Can you work these out from the drawing? Everything is in mm from the part's minimum corner. Coordinates: 2 decimals unless noted, no trailing zeros. Write each loop counter-clockwise with the first axis right and the second up, starting at its lowest first coordinate (ties: lowest second). Pieces come first, ordered by that corner, then holes. Notation, with made-up numbers: M -3,64 L 11,64 A22 ccw 11,81 Z; hole C 21.25,62.25 d11. An arc over 180 degrees is marked long. Write each question's results on one line, items separated by ' | '. Start each with the question number.
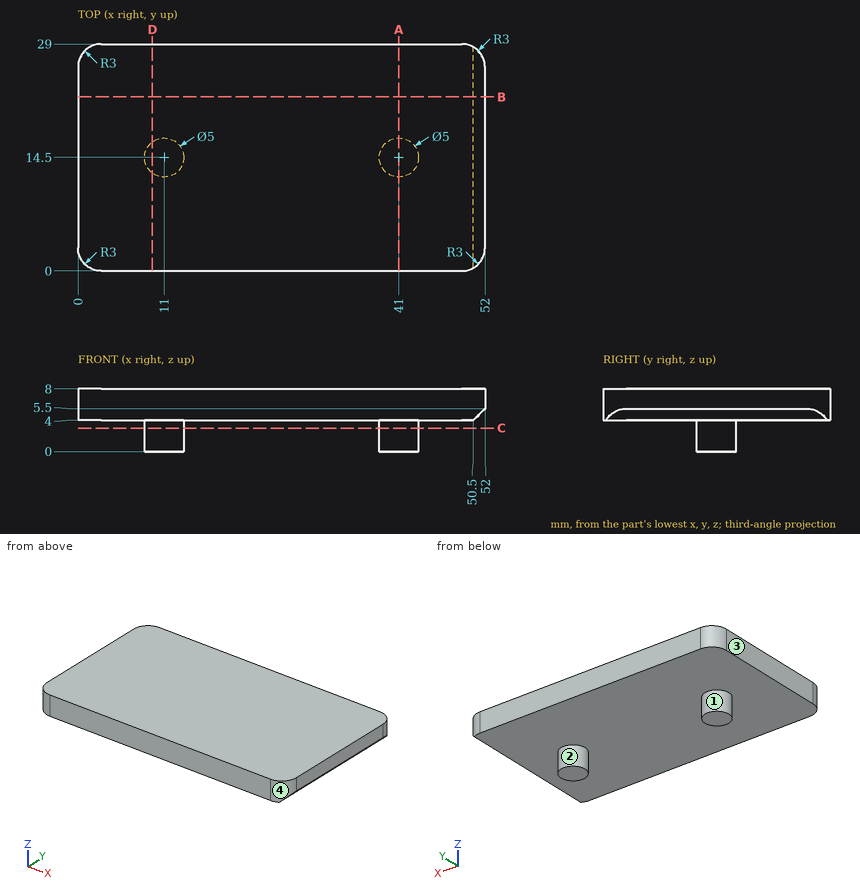
1) I want a section at D-D, the plane x = 9.5. Write out the boundary of the cut face in (y, z).
2) We'd pull the mould along X, two halves only. Please class the marked faces 1, 2, 3 and 4: pulls with the +X half, pulls with the -X half, needs draft (parallel to the pull), parting line crosses it, or undercut.
3) For pin 1 Ø4 at (x, y) = (30, 22.5) entering from -Z; pin 2 Ø3 at (y, z) = (24, 1.5) entering from -X (3 decimals); pin 3 Ø12 at (x, y) = (39.5, 20) entering from -Z, each with a flat end and sliding along its axis, tell me the tip position at first contact or that it passes through.
4) I want a section at B-B, the plane y = 22.25. Write out the boundary of the cut face in (x, z), then the cut area to 3 significant figures.
5) I want a section at C-C, the plane z = 3. Write out the boundary of the cut face in (x, y), then the cut area to 3 significant figures.
6) Please list where these lines run through material, in increasing order: line 1 (Z direction, x = 24, y = 19.5); line 2 (X direction, y = 16.5, z = 3.75); line 3 (X direction, y = 1, z = 5.5). Write a range as [from, to].
7) I want a section at A-A, the plane x = 41. Write out the boundary of the cut face in (y, z), then the cut area to 3 significant figures.
Output:
1) outline: M 0,4 L 12.5,4 L 12.5,0 L 16.5,0 L 16.5,4 L 29,4 L 29,8 L 0,8 Z
2) face 1: undercut | face 2: undercut | face 3: pulls with the -X half | face 4: pulls with the +X half
3) pin 1: stops at z = 4 | pin 2: passes through | pin 3: stops at z = 0
4) outline: M 0,4 L 50.5,4 L 52,5.5 L 52,8 L 0,8 Z | area: 207 mm2
5) outline: C 11,14.5 d5; C 41,14.5 d5 | area: 39.3 mm2
6) line 1: z = [4, 8] | line 2: x = [9.5, 12.5], [39.5, 42.5] | line 3: x = [0.76, 51.24]
7) outline: M 0,4 L 12,4 L 12,0 L 17,0 L 17,4 L 29,4 L 29,8 L 0,8 Z | area: 136 mm2
